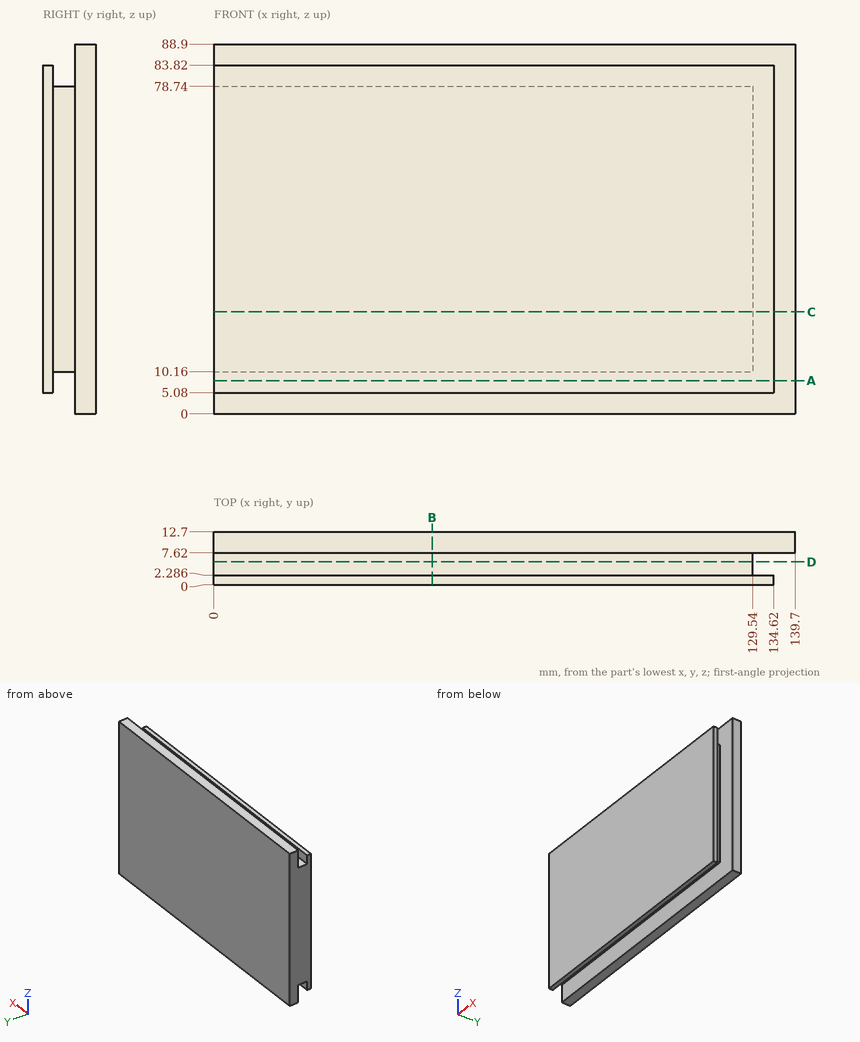
Geometry: see drawing. Coordinates: mm, zero at the bounding-box minimum. Give positions to 0.01 mm unless a question says otherwise; leave off trailing zeros. Write each loop counter-clockwise with the first axis right and the second up, starting at its lowest first coordinate (ties: lowest second). Pieces come first, ordered by that corner, then holes. Notation, with made-up numbers: (58, 55) -> (101, 55) arc R24 cw to (101, 67) -> close; hole circle Ø1 at (31, 70.5). An arc over 180 degrees is marked (long way). Use one line per item in the form item = value. Start each with the question number.
1) Ray query, probe 1 along Y at (x, z) = (7, 5.5); probe 2 along Z at (x, y) = (90.5, 2); probe 3 along Z at (x, y) = (125.5, 7). Return the intervals inside material, ascending. Write a range as from..to.
2) Pin query (flat end, axial travel): pin 1 (4 mm diameter, centred on x = 89, y = 4, fed in from +Z); pin 2 (5 mm diameter, centred on x = 66.5, y = 3.5, fed in from -Z); pin 3 (0.7 mm diameter, centred on y = 1, z = 42, fed in from +X). Return the tip coordinate at first contact, or that it passes through.
3) Section query A-A on z = 8. Return the cut outline in (x, y).
4) Section query B-B on x = 52.5. Return the cut outline in (y, z).
5) Section query D-D on y = 5.5. Return the cut outline in (x, z).
6) Section query C-C on z = 24.5. Return the cut outline in (x, y), then the cut area to 3 significant figures.
Outcome:
q1.probe_1 = 0..2.29, 7.62..12.7
q1.probe_2 = 5.08..83.82
q1.probe_3 = 10.16..78.74
q2.pin_1 = 83.82
q2.pin_2 = 5.08
q2.pin_3 = 134.62
q3.outline = (0, 0) -> (134.62, 0) -> (134.62, 2.29) -> (0, 2.29) -> close; (0, 7.62) -> (139.7, 7.62) -> (139.7, 12.7) -> (0, 12.7) -> close
q4.outline = (0, 5.08) -> (2.29, 5.08) -> (2.29, 10.16) -> (7.62, 10.16) -> (7.62, 0) -> (12.7, 0) -> (12.7, 88.9) -> (7.62, 88.9) -> (7.62, 78.74) -> (2.29, 78.74) -> (2.29, 83.82) -> (0, 83.82) -> close
q5.outline = (0, 10.16) -> (129.54, 10.16) -> (129.54, 78.74) -> (0, 78.74) -> close
q6.outline = (0, 0) -> (134.62, 0) -> (134.62, 2.29) -> (129.54, 2.29) -> (129.54, 7.62) -> (139.7, 7.62) -> (139.7, 12.7) -> (0, 12.7) -> close
q6.area = 1,710 mm^2
